Build history of the part. All positions in model axes, mm. Face numbers are marked on the shaded views. A direction names the side the tool comes from. Round coordinates to 2 decimals unless told otherwise and drop trailing zeros. Write each loop counter-clockwise with the first axis right and the second up, starting at its lowest first coordinate (ties: lowest second). Pieces come first, ordered by that corner, then holes. Notation, with made-up numbers: (73, -21) -> (99, -21) arc R21 cw to (99, -6) -> close; hole circle Ø5 at (71, 19). An arc over 180 degrees is marked (long way). Return JSON: item names as keys, results as strings.
from build123d import *

# Parameters (mm, degrees)
BOX_W             = 20
BOX_H             = 10
BOX_DEPTH         = 10
ARRAY_COUNT       = 6
CYLINDER001_R     = 20
CYLINDER001_DEPTH = 20
CYLINDER_R        = 30
CYLINDER_DEPTH    = 90


with BuildPart() as array_almenas:
    # Box → Box (new body)
    with BuildSketch(Plane(origin=(15, -5, 80), x_dir=(1, 0, 0), z_dir=(0, 0, 1))):
        with Locations((10, 5)):
            Rectangle(BOX_W, BOX_H)
    extrude(amount=BOX_DEPTH)

    # Array: Array_almenas ×6 about axis
    array_axis = Axis((0, 0, 0), (0, 0, 1))


with BuildPart() as array_almenas_1:
    add(array_almenas.part)
    for i in range(1, ARRAY_COUNT):
        add(array_almenas.part.rotate(array_axis, i * 360 / ARRAY_COUNT))


with BuildPart() as vaciadotorre:
    # Cylinder001 → Cylinder001 (new body)
    with BuildSketch(Plane.XY.offset(70)):
        Circle(CYLINDER001_R)
    extrude(amount=CYLINDER001_DEPTH)


with BuildPart() as obj1:
    # Cylinder → Cylinder (new body)
    with BuildSketch(Plane.XY):
        Circle(CYLINDER_R)
    extrude(amount=CYLINDER_DEPTH)

    # Cut: cut VaciadoTorre
    add(vaciadotorre.part, mode=Mode.SUBTRACT)

    # Cut001: cut Array_almenas
    add(array_almenas_1.part, mode=Mode.SUBTRACT)


solid = obj1.part
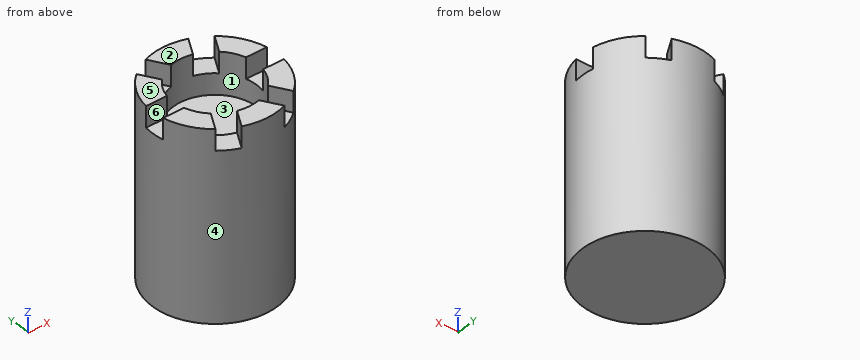
Q1. 3-axis set-ups, long thin cutter, end or side, ignore diameter. For the marked faces 5 and 6: which of +Z, -Z, +X, -X, +Y, -Y reach the whole face in a straight line?
Verdict:
{"face 5": "+Z, +X, -X, +Y, -Y", "face 6": "+Z, +X, -X"}
Q2. Saw through at B-B on z = 74.5. List the corners of the cut face in (x, y).
Verdict:
{"outline": "circle Ø60 at (0, 0); hole circle Ø40 at (0, 0)"}
Q3. Saw through at A-A on x = 0. List the corners of the cut face in (y, z), then the cut area to 3 significant figures.
Verdict:
{"outline": "(-30, 0) -> (30, 0) -> (30, 90) -> (20, 90) -> (20, 70) -> (-20, 70) -> (-20, 90) -> (-30, 90) -> close", "area": "4,600 mm²"}
Q4. Saw through at C-C on y = 0. List the corners of the cut face in (x, z).
Verdict:
{"outline": "(-30, 0) -> (30, 0) -> (30, 80) -> (20, 80) -> (20, 70) -> (-20, 70) -> (-20, 80) -> (-30, 80) -> close"}
Q5. Two-plate mould, pull along X, no slides. Class the marked faces 1, 2, 3 and 4: +X half, -X half, draft (parallel to the pull), parting line (faces both ways), or undercut.
Verdict:
{"face 1": "undercut", "face 2": "draft", "face 3": "undercut", "face 4": "parting line"}
Q6. Saw through at D-D on z = 65. List the corners of the cut face in (x, y), then the cut area to 3 significant figures.
Verdict:
{"outline": "circle Ø60 at (0, 0)", "area": "2,830 mm²"}
Q7. Pin check, flat tips, straight feed: pin 1 Ø3 at (x, y) = (-22, 0) entering from +Z; pin 2 Ø1 at (y, z) = (-17.5, 75.5) entering from +X; pin 3 Ø5 at (x, z) = (-15, 22.5) entering from +Y. Stop position of each tip, or through.
Verdict:
{"pin 1": "stops at z = 80", "pin 2": "stops at x = 24.72", "pin 3": "stops at y = 27.27"}
Q8. Wall check: L1, parallel to Y at x = 0, z = 80; L2, parallel to Z at x = 2.5, y = -2.5; L3, parallel to Y at x = -23, z = 84.5. Give the ranges that are in metal, low to high.
Verdict:
{"L1": "y = -30 to -20, 20 to 30", "L2": "z = 0 to 70", "L3": "y = -19.26 to -5, 5 to 19.26"}
